Source: CAD feature listing. Evaluate the final solid. Frame: model axes, mm. Face numbers are marked on the shaded views. A direction names the side the tool comes from. Coordinates: 2 decimals unless noted, no trailing zeros. Order: outer loops, then holes, each group sorted by start corner. A loop starts at its lowest first (then second) coordinate and runs counter-clockwise, first axis right, second up.
Item 1: Section C-C on x = 10.5. Return the cut outline in (y, z).
Item 2: Reachability of the marked faces 3 and 4 from +Z, -Z, +X, -X, +Y, -Y: full face, straight path, thin tool, end or side. Return the list, or none.
Item 3: Section A-A on x = 28.5. Return the cut outline in (y, z).
Item 4: Contact query for flat-ended pins moving along their axis: P1, Ø1.6, axis at x = 34, y = 3, coming from the -Z side; P2, Ø0.6, axis at x = -2.5, z = 5.5, coming from the +Y side; P3, Ø0.6, axis at y = -0.5, z = 5.5, coming from the +X side. Output: stop coordinate, or through.
Item 5: Section B-B on z = -7.5. Return the cut outline in (x, y).
Item 6: Mould query, pull axis Z, two halves, no side actions, for the marked faces 1 and 2. Classes: released by +Z, released by -Z, zero draft, split by the parting line, or undercut.
Item 7: Ray query, line 1 (Z direction, x = -33.5, y = 2.5); line 2 (X direction, y = 1.4, z = 0); line 3 (Y direction, x = -33.5, z = -7.25). Return the intervals inside material, ascending.
from build123d import *

# Parameters (mm, degrees)
SALIENTE_EXTRUIR1_DEPTH = 10.5
CORTAR_EXTRUIR1_DEPTH   = 48.9869774
ENVOLVER1_OUTLINE_W     = 4.5
ENVOLVER1_OUTLINE_H     = 1.5
ENVOLVER1_OUTLINE_W_2   = 6.094706288
ENVOLVER1_OUTLINE_H_2   = 1.606152826
ENVOLVER1_DEPTH         = 2
ENVOLVER1_START         = -3.5
ENVOLVER1_2_OUTLINE_W   = 25
ENVOLVER1_2_OUTLINE_H   = 2
ENVOLVER1_2_OUTLINE_H_2 = 1.5
ENVOLVER1_2_DEPTH       = 2
CROQUIS5_R              = 1.5
CORTAR_EXTRUIR2_DEPTH   = 48.9869774


# Read off the part's stored shape, not the designer's step: Envolver1
with BuildPart() as part:
    # Croquis1 → Saliente-Extruir1 (new, symmetric)
    with BuildSketch(Plane.XY):
        Polygon((-46.5, 2), (-46.5, 0), (-16.419869845, 0), (-13.785714286, 0), (-15.5, 2), align=None)
        Polygon((-13.785714286, 0), (-16.419869845, 0), (-13.419869845, -3.5), (13.419869845, -3.5), (16.419869845, 0), (13.785714286, 0), (12.5, -1.5), (-12.5, -1.5), align=None)
        Polygon((15.5, 2), (13.785714286, 0), (16.419869845, 0), (46.5, 0), (46.5, 2), align=None)
    extrude(amount=SALIENTE_EXTRUIR1_DEPTH, both=True)

    # Croquis3 → Cortar-Extruir1 (cut, through all)
    with BuildSketch(Plane(origin=(0, 2, 0), x_dir=(1, 0, 0), z_dir=(0, 1, 0))):
        with BuildLine():
            Line((-43.833986837, -4.5), (-43.5, -4.5))
            Line((-43.5, -4.5), (-43.5, -3))
            ThreePointArc((-43.5, -3), (-46.5, 0), (-43.5, 3))
            Line((-43.5, 3), (-43.5, 4.5))
            Line((-43.5, 4.5), (-43.833986837, 4.5))
            ThreePointArc((-43.833986837, 4.5), (-44.833986837, 5.5), (-43.833986837, 6.5))
            Line((-43.833986837, 6.5), (-43.5, 6.5))
            Line((-43.5, 6.5), (-43.5, 10.5))
            Line((-43.5, 10.5), (-43.5, 12.222660865))
            Line((-43.5, 12.222660865), (-52.324213339, 12.222660865))
            Line((-52.324213339, 12.222660865), (-52.324213339, -12.147175549))
            Line((-52.324213339, -12.147175549), (-43.5, -12.147175549))
            Line((-43.5, -12.147175549), (-43.5, -10.5))
            Line((-43.5, -10.5), (-43.5, -6.5))
            Line((-43.5, -6.5), (-43.833986837, -6.5))
            ThreePointArc((-43.833986837, -6.5), (-44.833986837, -5.5), (-43.833986837, -4.5))
        make_face()
        with BuildLine():
            Line((43.5, 12.222660865), (43.5, 10.5))
            Line((43.5, 10.5), (43.5, 6.5))
            Line((43.5, 6.5), (43.833986837, 6.5))
            ThreePointArc((43.833986837, 6.5), (44.833986837, 5.5), (43.833986837, 4.5))
            Line((43.833986837, 4.5), (43.5, 4.5))
            Line((43.5, 4.5), (43.5, 3))
            ThreePointArc((43.5, 3), (46.5, 0), (43.5, -3))
            Line((43.5, -3), (43.5, -4.5))
            Line((43.5, -4.5), (43.833986837, -4.5))
            ThreePointArc((43.833986837, -4.5), (44.833986837, -5.5), (43.833986837, -6.5))
            Line((43.833986837, -6.5), (43.5, -6.5))
            Line((43.5, -6.5), (43.5, -10.5))
            Line((43.5, -10.5), (43.5, -12.147175549))
            Line((43.5, -12.147175549), (52.324213339, -12.147175549))
            Line((52.324213339, -12.147175549), (52.324213339, 12.222660865))
            Line((52.324213339, 12.222660865), (43.5, 12.222660865))
        make_face()
    extrude(amount=-CORTAR_EXTRUIR1_DEPTH, mode=Mode.SUBTRACT)

    # Envolver1 outline → Envolver1 (add)
    with BuildSketch(Plane(origin=(0, 2, 0), x_dir=(1, 0, 0), z_dir=(0, 1, 0))):
        with BuildLine():
            Line((-15.5, -4.5), (-43.833986837, -4.5))
            ThreePointArc((-43.833986837, -4.5), (-44.833986837, -5.5), (-43.833986837, -6.5))
            Line((-43.833986837, -6.5), (-15.5, -6.5))
            Line((-15.5, -6.5), (-15.5, -4.5))
        make_face()
        with BuildLine():
            Line((43.833986837, -4.5), (15.5, -4.5))
            Line((15.5, -4.5), (15.5, -6.5))
            Line((15.5, -6.5), (43.833986837, -6.5))
            ThreePointArc((43.833986837, -6.5), (44.833986837, -5.5), (43.833986837, -4.5))
        make_face()
        with BuildLine():
            Line((-15.5, 6.5), (-43.833986837, 6.5))
            ThreePointArc((-43.833986837, 6.5), (-44.833986837, 5.5), (-43.833986837, 4.5))
            Line((-43.833986837, 4.5), (-15.5, 4.5))
            Line((-15.5, 4.5), (-15.5, 6.5))
        make_face()
        with BuildLine():
            Line((43.833986837, 6.5), (15.5, 6.5))
            Line((15.5, 6.5), (15.5, 4.5))
            Line((15.5, 4.5), (43.833986837, 4.5))
            ThreePointArc((43.833986837, 4.5), (44.833986837, 5.5), (43.833986837, 6.5))
        make_face()
        with Locations((17.75, 0)):
            Rectangle(ENVOLVER1_OUTLINE_W, ENVOLVER1_OUTLINE_H)
        with Locations((-17.75, 0)):
            Rectangle(ENVOLVER1_OUTLINE_W, ENVOLVER1_OUTLINE_H)
        with Locations((35, 0)):
            Rectangle(ENVOLVER1_OUTLINE_W_2, ENVOLVER1_OUTLINE_H_2)
        with Locations((-35, 0)):
            Rectangle(ENVOLVER1_OUTLINE_W_2, ENVOLVER1_OUTLINE_H_2)
    extrude(amount=ENVOLVER1_DEPTH)

    # Envolver1 2 outline → Envolver1 2 (add)
    with BuildSketch(Plane(origin=(0, 2, 0), x_dir=(1, 0, 0), z_dir=(0, 1, 0)).offset(ENVOLVER1_START)):
        with Locations((0, -5.5)):
            Rectangle(ENVOLVER1_2_OUTLINE_W, ENVOLVER1_2_OUTLINE_H)
        with Locations((0, 5.5)):
            Rectangle(ENVOLVER1_2_OUTLINE_W, ENVOLVER1_2_OUTLINE_H)
        Rectangle(ENVOLVER1_2_OUTLINE_W, ENVOLVER1_2_OUTLINE_H_2)
    extrude(amount=ENVOLVER1_2_DEPTH)

    # Croquis5 → Cortar-Extruir2 (cut, through all)
    with BuildSketch(Plane(origin=(0, 2, 0), x_dir=(1, 0, 0), z_dir=(0, 1, 0))):
        with Locations(Location((-42.5, 0, 0), (0, 0, 270))):
            Circle(CROQUIS5_R)
        with Locations(Location((42.5, 0, 0), (0, 0, 270))):
            Circle(CROQUIS5_R)
        with Locations(Location((28.5, 0, 0), (0, 0, 270))):
            Circle(CROQUIS5_R)
        with Locations(Location((-28.5, 0, 0), (0, 0, 270))):
            Circle(CROQUIS5_R)
    extrude(amount=-CORTAR_EXTRUIR2_DEPTH, mode=Mode.SUBTRACT)


solid = part.part
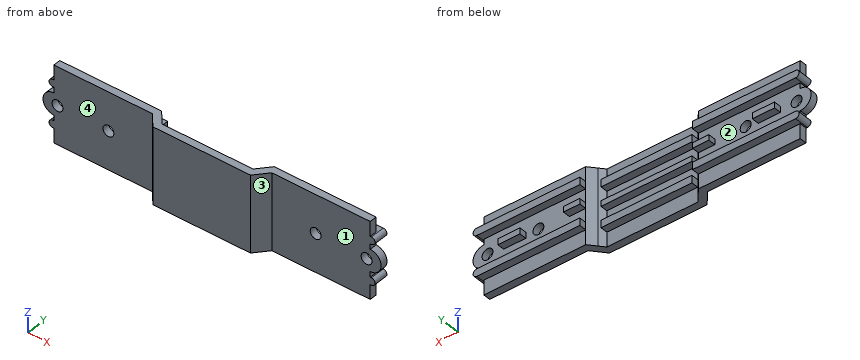
Answer list:
1. outline: (-3.5, -10.5) - (-1.5, -10.5) - (-1.5, -6.5) - (0.5, -6.5) - (0.5, -4.5) - (-1.5, -4.5) - (-1.5, -0.75) - (0.5, -0.75) - (0.5, 0.75) - (-1.5, 0.75) - (-1.5, 4.5) - (0.5, 4.5) - (0.5, 6.5) - (-1.5, 6.5) - (-1.5, 10.5) - (-3.5, 10.5) - close
2. face 3: +Z, -Z, +X, -Y
2. face 4: +Z, -Z, -X, -Y
3. outline: (0, -10.5) - (2, -10.5) - (2, -6.5) - (4, -6.5) - (4, -4.5) - (2, -4.5) - (2, -1.5) - (0, -1.5) - close; (0, 1.5) - (2, 1.5) - (2, 4.5) - (4, 4.5) - (4, 6.5) - (2, 6.5) - (2, 10.5) - (0, 10.5) - close
4. P1: stops at z = -6.5
4. P2: stops at y = 0.5
4. P3: stops at x = 16.25
5. outline: (-43.5, 0) - (-16.42, 0) - (-13.42, -3.5) - (13.42, -3.5) - (16.42, 0) - (43.5, 0) - (43.5, 2) - (15.5, 2) - (12.5, -1.5) - (-12.5, -1.5) - (-15.5, 2) - (-43.5, 2) - close
6. face 1: zero draft
6. face 2: undercut
7. line 1: z = -6.5 to -4.5, -0.8 to 0.8, 4.5 to 6.5
7. line 2: x = -46.5 to -44, -41 to -30, -27 to -14.99, 14.99 to 27, 30 to 41, 44 to 46.5
7. line 3: y = 0 to 2
